Geometry check sheet. Reference: the model listing, model coordinates, mm. A direction names the side the tool comes from. Give positions to 0.01 mm unless a question says otherwise; leave off trailing zeros. Loops run counter-clockwise (first coordinate to the right, second up) from the corner with the lowest first, then second, coordinate; pieces in that order, holes last. Notation, with made-up numbers: (72, -3) -> (126, -3) arc R21 ccw to (126, 18) -> close; hole circle Ø11 at (53, -28.75). An arc over 180 degrees is marked (long way). Answer as a JSON object with one key per item and string values.
Autodesk Inventor part; units mm, degrees
ref_plane "YZ Plane" through (0, 0, 0) normal (1, 0, 0) x (0, 1, 0)
ref_plane "XZ Plane" through (0, 0, 0) normal (0, 1, 0) x (-1, 0, 0)
ref_plane "XY Plane" through (0, 0, 0) normal (0, 0, 1) x (1, 0, 0)
sketch "Boceto1" plane through (0, 0, 0) normal (0, 1, 0) x (-1, 0, 0)
  line L0 (0.0239, -45) -> (35.0239, -45)
  line L1 (35.0239, -10) -> (-34.9761, -10)
  line L2 (-40.6213, -10) -> (-84.6707, -10)
  line L3 (-100, -10) -> (100, -10)
  line L4 (-100, -10) -> (100, -10)
  line L5 (105.0239, -10) -> (-104.9761, -10)
  line L6 (105.0239, -10) -> (-104.9761, -10)
  line L7 (105, 10) -> (-105, 10)
  line L8 (105, 10) -> (-105, 10)
  line L9 (0.0239, -45) -> (-34.9761, -45)
  circle A0 centre (11.5239, -60) radius 3
  circle A1 centre (11.5239, -30) radius 3
  circle A2 centre (-11.4761, -30) radius 3
  line L10 (11.5239, -30) -> (-11.4761, -60)
  line L11 (-34.9761, -79) -> (35.0239, -79)
  line L12 (-34.9761, -10) -> (-34.9761, -79)
  circle A3 centre (-11.4761, -60) radius 3
  line L13 (11.5239, -60) -> (-11.4761, -30)
  line L14 (35.0239, -45) -> (35.0239, -10)
  line L15 (35.0239, -79) -> (35.0239, -10)
  point P0 (0, 0)
  point P1 (0, 0)
  point P2 (0, 0)
  point P3 (0.0478, -10)
  point P4 (0, 0)
  point P5 (-95.8154, 10)
  dimension "d0" = 20
  dimension "d1" = 20
  dimension "d2" = 30
  dimension "d3" = 30
  dimension "d4" = 20
  dimension "d5" = 35
  dimension "d6" = 35
  dimension "d7" = 69
extrude "Extrusión1" add sketch "Boceto1" along normal blind 10
sketch "Boceto2" plane through (0, 0, 0) normal (0, -1, 0) x (1, 0, 0)
  line L0 (-35.0239, -10) -> (34.9761, -10)
  line L1 (-35.0239, -10) -> (-35.0239, 50)
  line L2 (-35.0239, 50) -> (34.9761, 50)
  line L3 (34.9761, 50) -> (34.9761, -10)
  point P0 (0, 0)
  dimension "d10" = 60
extrude "Extrusión2" add sketch "Boceto2" against normal blind 50
sketch "Boceto3" plane through (0, 50, 0) normal (0, 1, 0) x (1, 0, 0)
  line L0 (-35.0239, 79) -> (-35.0239, -50)
  line L1 (-35.0239, 9.9865) -> (-35.0239, -50)
  line L2 (-11, -45.0068) -> (11, -45.0068)
  line L3 (11, -45.0068) -> (11, 4.9932)
  line L4 (11, 4.9932) -> (-11, 4.9932)
  line L5 (-11, 4.9932) -> (-11, -45.0068)
  line L6 (-11, -45.0068) -> (11, 4.9932) construction
  line L7 (11, -45.0068) -> (-11, 4.9932) construction
  point P0 (0, 0)
  point P1 (0, -20.0068)
  dimension "d13" = 22
  dimension "d14" = 50
extrude "Extrusión3" cut sketch "Boceto3" against normal blind 43
ref_plane "Plano de trabajo1" through (-0.0239, 0, -79) normal (-1, 0, 0) x (0, 0, 1)
sketch "Boceto4" plane through (-0.0239, 0, -79) normal (-1, 0, 0) x (0, 0, 1)
  line L0 (69, 10) -> (0, 10)
  line L1 (69, 10) -> (40.4098, 10)
  line L2 (69, 10) -> (69, 50)
  line L3 (69, 10) -> (69, 42.6104)
  line L4 (69, 35.4459) -> (55.8036, 8.5042)
  point P0 (79, 0)
  point P1 (56.5363, 10)
  dimension "d17" = 30
extrude "Extrusión4" add sketch "Boceto4" along normal mid plane 15
properties part number "servo_piece"
1) Section check B-B on z = -60. Record the cut outline in (x, y), plus the area to 3 significant figures.
Geometry check:
{"outline": "(-35.02, 0) -> (-14.52, 0) -> (-14.52, 10) -> (-35.02, 10) -> close; (-8.52, 0) -> (8.48, 0) -> (8.48, 10) -> (-8.52, 10) -> close; (14.48, 0) -> (34.98, 0) -> (34.98, 10) -> (14.48, 10) -> close", "area": "580 mm2"}
2) Section check C-C on x = -1. Record the cut outline in (y, z), plus the area to 3 significant figures.
Geometry check:
{"outline": "(0, -79) -> (10, -79) -> (10, -22.46) -> (35.45, -10) -> (50, -10) -> (50, -4.99) -> (7, -4.99) -> (7, 45.01) -> (50, 45.01) -> (50, 50) -> (0, 50) -> close", "area": "1,700 mm2"}
3) Section check A-A on y = 8.5. Record the cut outline in (x, z), plus the area to 3 significant figures.
Geometry check:
{"outline": "(-35.02, -79) -> (34.98, -79) -> (34.98, 50) -> (-35.02, 50) -> close; hole circle Ø6 at (-11.52, -60); hole circle Ø6 at (-11.52, -30); hole (-11, -4.99) -> (11, -4.99) -> (11, 45.01) -> (-11, 45.01) -> close; hole circle Ø6 at (11.48, -60); hole circle Ø6 at (11.48, -30)", "area": "7,820 mm2"}
4) Tool access check on faces 1 (the face through (11, 29, 20)), 2 (the face through (0, 5, -79)). Record the directions out of +Z, -Z, +X, -X, +Y, -Y that give a thin tool (end or side, any length) a straight path to the whole face; none if there is none.
Geometry check:
{"face 1": "+Y", "face 2": "-Z, +X, -X, +Y, -Y"}
5) Material ranges on line 1 along Z through (x, y) = (-10.5, 43.5); line 2 along X through (y, z) = (16.5, 26); line 3 along Y through (x, z) = (-31, -53.5), recorded low to high. Write a range as from..to.
Geometry check:
{"line 1": "z = -10..-4.99, 45.01..50", "line 2": "x = -35.02..-11, 11..34.98", "line 3": "y = 0..10"}
6) Section check D-D on z = 28. Record the cut outline in (x, y), plus the area to 3 significant figures.
Geometry check:
{"outline": "(-35.02, 0) -> (34.98, 0) -> (34.98, 50) -> (11, 50) -> (11, 7) -> (-11, 7) -> (-11, 50) -> (-35.02, 50) -> close", "area": "2,550 mm2"}
7) Draft check along X on faces 3 (the face through (-16, 50, 20)), 4 (the face through (14.473, 4.93, -30.132)), 5 (the face through (-35.024, 19, 13)), 6 (the face through (7.476, 17, -14)). Enter one of: pulls with the +X half, pulls with the -X half, needs draft (parallel to the pull), parting line crosses it, or undercut.
Geometry check:
{"face 3": "needs draft", "face 4": "undercut", "face 5": "pulls with the -X half", "face 6": "pulls with the +X half"}
8) Depth check by flat-ended pin: P1, Ø9.5, axis at x = 11.48, z = -60, coming from the -Y side; P2, Ø3.5, axis at y = 17.5, z = -16.5, coming from the +X side; P3, Ø12, axis at x = -15.5, y = 36, coming from the -Z side; P4, Ø20.5, axis at x = 10.5, z = -51.5, coming from the +Y side. Enter the tip coordinate at first touch or a pass-through.
Geometry check:
{"P1": "stops at y = 0", "P2": "stops at x = 7.48", "P3": "stops at z = -10", "P4": "stops at y = 10"}
